from build123d import *

# Parameters (mm, degrees)
F1_DEPTH = 12.7
F3_DEPTH = 38.1
F4_W     = 31.75
F4_H     = 14.2875
F5_DEPTH = 38.1
F6_R     = 6.35
F7_DEPTH = 14.2875


with BuildPart() as f1:
    # F0 (on Front) → F1 (new body)
    with BuildSketch(Plane.XZ):
        Polygon((-74.188948, 10.506319), (-74.188948, -11.718681), (52.811052, -11.718681), (52.811052, 10.506319), (5.186052, 58.131319), (-26.563948, 58.131319), align=None)
    extrude(amount=F1_DEPTH)

    # F2 (on Front) → F3 (join)
    with BuildSketch(Plane.XZ):
        Polygon((-42.438948, 0.981418), (-42.438948, -11.718582), (21.061052, -11.718582), (21.061052, 0.981418), (2.011052, 20.031418), (-23.388948, 20.031418), align=None)
    extrude(amount=F3_DEPTH)

    # F4 (on Front) → F5 (join)
    with BuildSketch(Plane.XZ):
        with Locations((-10.846151, 50.999742)):
            Rectangle(F4_W, F4_H)
    extrude(amount=F5_DEPTH)

    # F6 (on face) → F7 (cut)
    with BuildSketch(Plane.XY.offset(58.143492)):
        with Locations((-10.846151, -22.225)):
            Circle(F6_R)
    extrude(amount=-F7_DEPTH, mode=Mode.SUBTRACT)


solid = f1.part
Check sheet for the modelled part. Datum: model origin and axes. Units: mm. A direction names the side the tool comes from. Round coordinates to 2 decimals unless told otherwise and drop trailing zeros. Loops run counter-clockwise (first coordinate to the right, second up) from the corner with the lowest first, then second, coordinate; pieces in that order, holes last. Notation, with made-up numbers: (40, -18) - (64, -18) arc R30 ccw to (64, 7) - close; hole circle Ø8 at (-13.75, 86). An arc over 180 degrees is marked (long way). Answer as CSV lines item,"result". Start each with the question number.
Item 1: Depth check by flat-ended pin: P1, Ø1.5, axis at y = -29, z = 4, coming from the -X side; P2, Ø11.5, axis at y = -10, z = 52.5, coming from the -X side; P3, Ø11.5, axis at y = -19, z = 52, coming from the +X side. Enter the tip coordinate at first touch or a pass-through.
Item 2: Release check for a two-part mould opening along Z. For faces 4 (the flat face through (-7.5, -28, 43.856)), 5 (the flat face through (21.061, -25, -5)), 6 (the flat face through (-12, -6, -11.719)), 7 (the flat face through (29.33, -6.26, 33.99)) record: +Z half, -Z half, draft (parallel to the pull), parting line (faces both ways), or undercut.
Item 3: Section check A-A (y = -31.5). Record the boundary of the cut face in (x, z).
Item 4: Set-up check for faces 1 (the flat face through (-26.721, -27, 51)), 2 (the flat face through (5.029, -27, 51)), 3 (the flat face through (-32.78, -25.22, 10.64)): record each of +Z, -Z, +X, -X, +Y, -Y from which the full face is reachable in a straight line by a thin tool's end or side.
Item 5: Section check B-B (z = -1). Record the boundary of the cut face in (x, y).
Item 6: Scan lines: line 1 (Y direction, x = -32, z = 22); line 2 (X direction, y = -14, z = 45.5); line 3 (X direction, y = -23.5, z = 45). Record each from-to range of solid material in increasing order. Write a range as [from, to].
Report:
1,P1,"stops at x = -40.17"
1,P2,"stops at x = -37.95"
1,P3,"stops at x = 5.03"
2,face 4,"undercut"
2,face 5,"draft"
2,face 6,"-Z half"
2,face 7,"+Z half"
3,outline,"(-42.44, -11.72) - (21.06, -11.72) - (21.06, 0.98) - (2.01, 20.03) - (-23.39, 20.03) - (-42.44, 0.98) - close; (-26.72, 43.86) - (5.03, 43.86) - (5.03, 58.14) - (-26.72, 58.14) - close"
4,face 1,"+Z, -X, -Y"
4,face 2,"+Z, +X, -Y"
4,face 3,"-X, -Y"
5,outline,"(-74.19, -12.7) - (-42.44, -12.7) - (-42.44, -38.1) - (21.06, -38.1) - (21.06, -12.7) - (52.81, -12.7) - (52.81, 0) - (-74.19, 0) - close"
6,line 1,"y = [-12.7, 0]"
6,line 2,"x = [-26.72, 5.03]"
6,line 3,"x = [-26.72, -17.07], [-4.63, 5.03]"
